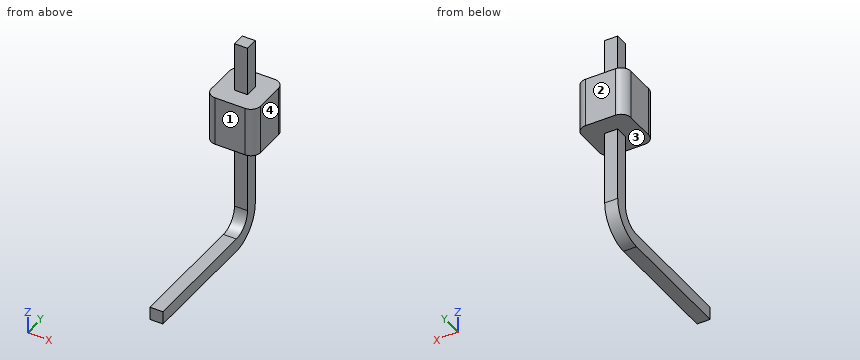
```python
from build123d import *

# Parameters (mm, degrees)
SKETCH_1_W      = 2.54
SKETCH_1_H      = 2.54
EXTRUDE_1_DEPTH = 2.54
SKETCH_2_W      = 0.67
SKETCH_2_H      = 0.67
FILLET_1_R      = 0.5


with BuildPart() as part:
    # 草图1 → 拉伸1 (new body)
    with BuildSketch(Plane.XY):
        with Locations((0, -1.289090726)):
            Rectangle(SKETCH_1_W, SKETCH_1_H)
    extrude(amount=EXTRUDE_1_DEPTH)

    # 扫描1: sweep along a path in 草图3
    with BuildLine(Plane(origin=(0, 0, 0), x_dir=(0, 0, -1), z_dir=(1, 0, 0))) as sweep_1_path:
        Line((-5.08, -1.299090726), (3.8, -1.299090726))
        ThreePointArc((3.8, -1.299090726), (4.70509668, -1.673994046), (5.08, -2.579090726))
        Line((5.08, -2.579090726), (5.08, -8.919090726))
    # 草图2 → 扫描1 (sweep)
    with BuildSketch(Plane(origin=(0, 0, 5.08), x_dir=(-1, 0, 0), z_dir=(0, 0, -1))):
        with Locations((0, -1.289090726)):
            Rectangle(SKETCH_2_W, SKETCH_2_H)
    sweep(path=sweep_1_path.line)

    # 圆角1
    fillet_1_edges = [part.edges().sort_by_distance(p)[0] for p in [
        (-1.27, -0.019090726, 1.27),
        (1.27, -0.019090726, 1.27),
        (1.27, -2.559090726, 1.27),
        (-1.27, -2.559090726, 1.27),
    ]]
    fillet(fillet_1_edges, radius=FILLET_1_R)


solid = part.part
```
Part model, mm, in its own coordinate system. Face numbers are marked on the shaded views. A direction names the side the tool comes from. Give positions to 0.01 mm unless a question says otherwise; leave off trailing zeros. Order: outer loops, then holes, each group sorted by start corner. A loop starts at its lowest first (then second) coordinate and runs counter-clockwise, first axis right, second up. Notation, with made-up numbers: M -36.5,6.5 L -30.5,6.5 A19 ccw -30.5,39.5 Z; hole C 66.25,5 d3. An arc over 180 degrees is marked long. Use a Markdown table: item, result. Add a question column.
(1) Drop flat-ended pins along their axis: P1, Ø2.5, axis at y = -6, z = -4, coming from the -X side (3 decimals); P2, Ø1, axis at x = -0.5, z = -2, coming from the +Y side; P3, Ø0.7, axis at y = -1, z = 4.5, coming from the +X side (3 decimals). Give the stop position or say it passes through.
(2) Saw through at B-B, the plane y = -1.75. Give the cut face in (x, z) (3 decimals).
(3) Saw through at A-A, the plane z = 2. Give the cut face in (x, y), and give its area (3 significant figures).
(4) 3-axis set-ups, long thin cutter, end or side, ignore diameter. For the marked faces 1 and 2: which of +Z, -Z, +X, -X, +Y, -Y reach the whole face in a straight line?
(5) Probe line 1 along Y through (x, z) = (-0.75, 2); line 2 along Z through (x, y) = (0.85, -0.75); line 3 along Y through (x, z) = (-0.3, -0.5). List the from-to ranges inside material, lowest first. Write a range as [from, to].
(6) Saw through at C-C, the plane x = -0.65. Give the cut face in (y, z), and give its area (3 significant figures).
(7) Mould opens along Z. For the marked faces 3 and 4 say: +Z half, -Z half, draft (parallel to the pull), parting line (faces both ways), or undercut.
(8) Saw through at D-D, the plane y = -5.5. Give the cut face in (x, z) (3 decimals), and give its area (3 significant figures).
Answer key:
| question | item | result |
|---|---|---|
| 1 | P1 | x = -0.335 |
| 1 | P2 | y = -0.95 |
| 1 | P3 | x = 0.335 |
| 2 | outline | M -1.27,0 L 1.27,0 L 1.27,2.54 L -1.27,2.54 Z; M -0.335,-5.198 L 0.335,-5.198 L 0.335,-4.274 L -0.335,-4.274 Z |
| 3 | outline | M -1.27,-2.06 A0.5 ccw -0.77,-2.56 L 0.77,-2.56 A0.5 ccw 1.27,-2.06 L 1.27,-0.52 A0.5 ccw 0.77,-0.02 L -0.77,-0.02 A0.5 ccw -1.27,-0.52 Z |
| 3 | area | 6.24 mm^2 |
| 4 | face 1 | +Z, +X, -X, -Y |
| 4 | face 2 | +Z, -Z, +X, -X, +Y |
| 5 | line 1 | [-2.56, -0.02] |
| 5 | line 2 | [0, 2.54] |
| 5 | line 3 | [-1.62, -0.95] |
| 6 | outline | M -2.56,0 L -0.02,0 L -0.02,2.54 L -2.56,2.54 Z |
| 6 | area | 6.45 mm^2 |
| 7 | face 3 | undercut |
| 7 | face 4 | draft |
| 8 | outline | M -0.335,-5.425 L 0.335,-5.425 L 0.335,-4.755 L -0.335,-4.755 Z |
| 8 | area | 0.449 mm^2 |
